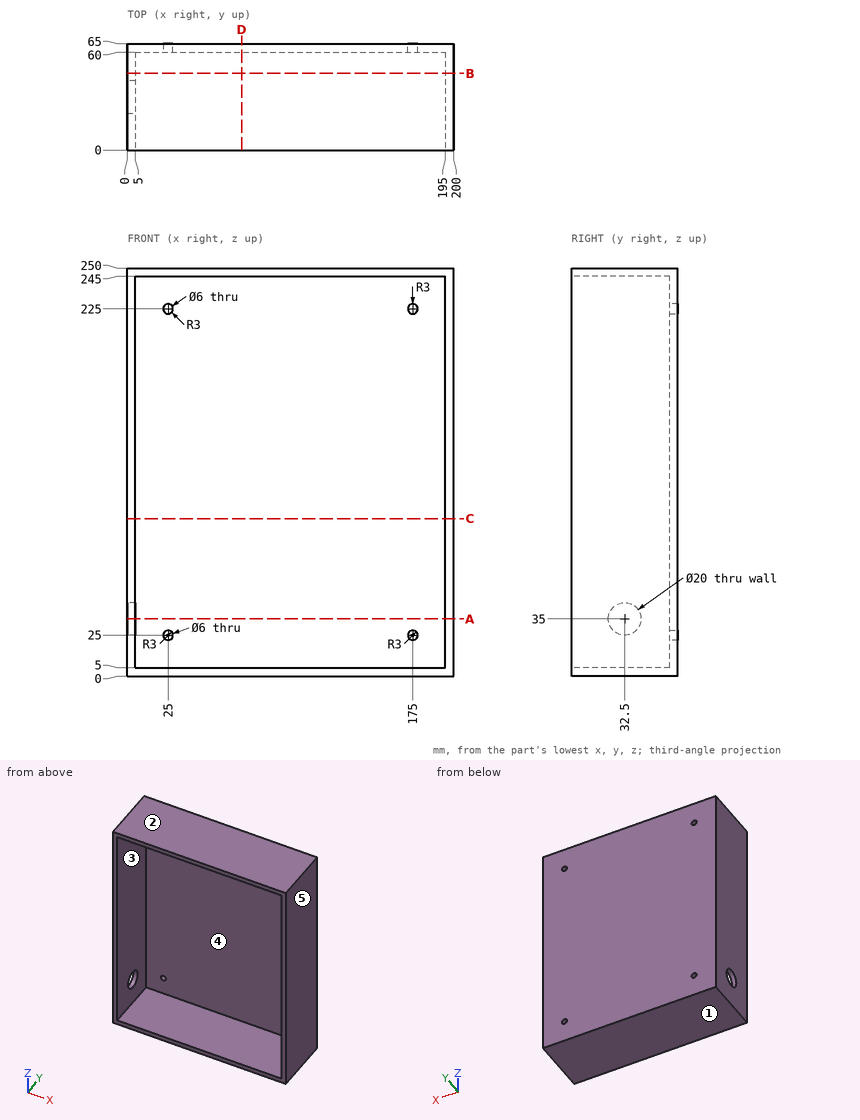
Could you check a few things on this drawing? It's one solid part, dimensions in mm from its lowest x, y, z. A direction names the side the tool comes from. Round coordinates to 2 decimals unless told otherwise and drop trailing zeros. Loops run counter-clockwise (first coordinate to the right, second up) from the corner with the lowest first, then second, coordinate; pieces in that order, holes last.
Q1. Thinking about a two-plate mould opening in Z: for the marked faces 1, 2 and 3, which applies, pulls with the +Z half, pulls with the -Z half, needs draft (parallel to the pull), parting line crosses it, or undercut?
Q2. I want a section at C-C (z = 96.5). Write out the boundary of the cut face in (x, y).
Q3. I want a section at B-B (y = 47). Write out the boundary of the cut face in (x, z).
Q4. For P1, Ø6, axis at x = 65, z = 146.5, coming from the -Y side; P2, Ø3.5, axis at x = 25, z = 225, coming from the -Y side; P3, Ø18, axis at y = 32.5, z = 35, coming from the -X side, each with a flat end and sliding along its axis, tell me the tip position at first contact or that it passes through.
Q5. I want a section at A-A (z = 35). Write out the boundary of the cut face in (x, y).
Q6. I want a section at D-D (x = 70). Write out the boundary of the cut face in (y, z), and give its area (3 significant figures).
Q7. Please list where these lines run through material, in increasing order: L1, parallel to Z at x = 49, y = 36; L2, parallel to X at y = 17, z = 169; L3, parallel to Y at x = 88, z = 125.
Q8. On a 3-axis mill with a long thin cutter (end or side, diameter ignored), from which of +Z, -Z, +X, -X, +Y, -Y can I reach the whole of each face in a straight line? I mean the marked faces 4 and 5. Say none if no direction works.
Answer below:
1. face 1: pulls with the -Z half
1. face 2: pulls with the +Z half
1. face 3: undercut
2. outline: (0, 0) - (5, 0) - (5, 60) - (195, 60) - (195, 0) - (200, 0) - (200, 65) - (0, 65) - close
3. outline: (0, 0) - (200, 0) - (200, 250) - (0, 250) - close; hole (5, 5) - (195, 5) - (195, 245) - (5, 245) - close
4. P1: stops at y = 60
4. P2: passes through
4. P3: stops at x = 195
5. outline: (0, 0) - (5, 0) - (5, 22.5) - (0, 22.5) - close; (0, 42.5) - (5, 42.5) - (5, 60) - (195, 60) - (195, 0) - (200, 0) - (200, 65) - (0, 65) - close
6. outline: (0, 0) - (65, 0) - (65, 250) - (0, 250) - (0, 245) - (60, 245) - (60, 5) - (0, 5) - close
6. area: 1,850 mm2
7. L1: z = 0 to 5, 245 to 250
7. L2: x = 0 to 5, 195 to 200
7. L3: y = 60 to 65
8. face 4: -Y
8. face 5: +Z, -Z, +X, +Y, -Y
